from build123d import *

# Parameters (mm, degrees)
BOSS_EXTRU_1_CORPS_DEPTH    = 110
CONG_1_R                    = 1.5
CONG_2_R                    = 0.4
CONG_4_R                    = 1
CONG_1_OF_SYM_TRIE_BRAS_R   = 1.5
CONG_2_OF_SYM_TRIE_BRAS_R   = 0.4
CONG_4_OF_SYM_TRIE_BRAS_R   = 1
SYM_TRIE_BRAS_DOUBLE_DEPTH  = 110
APR_S_TARODAGE_M6_R         = 3
ENL_V_MAT_FILETAGE_M6_DEPTH = 111.905365064


# Read off the part's stored shape, not the designer's step: Symétrie Bras double
with BuildPart() as part:
    # Esquisse4 → Boss.-Extru.1 Corps (new body)
    with BuildSketch(Plane(origin=(0, 0, 0), x_dir=(1, 0, 0), z_dir=(0, 1, 0))):
        Polygon((0, 0), (-4.5, 0), (-4.5, 3.625), (-6.875, 6), (-8.5, 6), (-8.5, 3), (-9.5, 3), (-9.5, 3.5), (-10, 3.5), (-10, 10), (-3.5, 10), (-3.5, 9.5), (-3, 9.5), (-3, 8.5), (-6, 8.5), (-6, 6.875), (-3.625, 4.5), (0, 4.5), align=None)
    boss_extru_1_corps = extrude(amount=BOSS_EXTRU_1_CORPS_DEPTH)

    # Congé1
    cong_1_edges = [part.edges().sort_by_distance(p)[0] for p in [
        (-10, 55, -10),
    ]]
    fillet(cong_1_edges, radius=CONG_1_R)

    # Congé2
    cong_2_edges = [part.edges().sort_by_distance(p)[0] for p in [
        (-8.5, 55, -6),
        (-6, 55, -8.5),
    ]]
    fillet(cong_2_edges, radius=CONG_2_R)

    # Congé4
    cong_4_edges = [part.edges().sort_by_distance(p)[0] for p in [
        (-4.5, 55, -3.625),
        (-6.875, 55, -6),
        (-6, 55, -6.875),
        (-3.625, 55, -4.5),
    ]]
    fillet(cong_4_edges, radius=CONG_4_R)

    # Symétrie Bras: Boss.-Extru.1 Corps across plane
    add(boss_extru_1_corps.mirror(Plane(origin=(0, 110, -4.5), x_dir=(0, 0, 1), z_dir=(-1, 0, 0))))

    # Congé1 of Symétrie Bras
    cong_1_of_sym_trie_bras_edges = [part.edges().sort_by_distance(p)[0] for p in [
        (10, 55, -10),
    ]]
    fillet(cong_1_of_sym_trie_bras_edges, radius=CONG_1_OF_SYM_TRIE_BRAS_R)

    # Congé2 of Symétrie Bras
    cong_2_of_sym_trie_bras_edges = [part.edges().sort_by_distance(p)[0] for p in [
        (8.5, 55, -6),
        (6, 55, -8.5),
    ]]
    fillet(cong_2_of_sym_trie_bras_edges, radius=CONG_2_OF_SYM_TRIE_BRAS_R)

    # Congé4 of Symétrie Bras
    cong_4_of_sym_trie_bras_edges = [part.edges().sort_by_distance(p)[0] for p in [
        (4.5, 55, -3.625),
        (6.875, 55, -6),
        (6, 55, -6.875),
        (3.625, 55, -4.5),
    ]]
    fillet(cong_4_of_sym_trie_bras_edges, radius=CONG_4_OF_SYM_TRIE_BRAS_R)

    # Symétrie Bras double outline → Symétrie Bras double (add)
    with BuildSketch(Plane(origin=(0, 0, 0), x_dir=(1, 0, 0), z_dir=(0, 1, 0))):
        with BuildLine():
            ThreePointArc((7.289213562, -6), (6.90653013, -5.923879533), (6.582106781, -5.707106781))
            Line((6.582106781, -5.707106781), (4.792893219, -3.917893219))
            ThreePointArc((4.792893219, -3.917893219), (4.576120467, -3.59346987), (4.5, -3.210786438))
            Line((4.5, -3.210786438), (4.5, 0))
            Line((4.5, 0), (-4.5, 0))
            Line((-4.5, 0), (-4.5, -3.210786438))
            ThreePointArc((-4.5, -3.210786438), (-4.576120467, -3.59346987), (-4.792893219, -3.917893219))
            Line((-4.792893219, -3.917893219), (-6.582106781, -5.707106781))
            ThreePointArc((-6.582106781, -5.707106781), (-6.90653013, -5.923879533), (-7.289213562, -6))
            Line((-7.289213562, -6), (-8.1, -6))
            ThreePointArc((-8.1, -6), (-8.382842712, -5.882842712), (-8.5, -5.6))
            Line((-8.5, -5.6), (-8.5, -3))
            Line((-8.5, -3), (-9.5, -3))
            Line((-9.5, -3), (-9.5, -3.5))
            Line((-9.5, -3.5), (-10, -3.5))
            Line((-10, -3.5), (-10, -8.5))
            ThreePointArc((-10, -8.5), (-9.560660172, -9.560660172), (-8.5, -10))
            Line((-8.5, -10), (-3.5, -10))
            Line((-3.5, -10), (-3.5, -9.5))
            Line((-3.5, -9.5), (-3, -9.5))
            Line((-3, -9.5), (-3, -8.5))
            Line((-3, -8.5), (-5.6, -8.5))
            ThreePointArc((-5.6, -8.5), (-5.882842712, -8.382842712), (-6, -8.1))
            Line((-6, -8.1), (-6, -7.289213562))
            ThreePointArc((-6, -7.289213562), (-5.923879533, -6.90653013), (-5.707106781, -6.582106781))
            Line((-5.707106781, -6.582106781), (-3.917893219, -4.792893219))
            ThreePointArc((-3.917893219, -4.792893219), (-3.59346987, -4.576120467), (-3.210786438, -4.5))
            Line((-3.210786438, -4.5), (3.210786438, -4.5))
            ThreePointArc((3.210786438, -4.5), (3.59346987, -4.576120467), (3.917893219, -4.792893219))
            Line((3.917893219, -4.792893219), (5.707106781, -6.582106781))
            ThreePointArc((5.707106781, -6.582106781), (5.923879533, -6.90653013), (6, -7.289213562))
            Line((6, -7.289213562), (6, -8.1))
            ThreePointArc((6, -8.1), (5.882842712, -8.382842712), (5.6, -8.5))
            Line((5.6, -8.5), (3, -8.5))
            Line((3, -8.5), (3, -9.5))
            Line((3, -9.5), (3.5, -9.5))
            Line((3.5, -9.5), (3.5, -10))
            Line((3.5, -10), (8.5, -10))
            ThreePointArc((8.5, -10), (9.560660172, -9.560660172), (10, -8.5))
            Line((10, -8.5), (10, -3.5))
            Line((10, -3.5), (9.5, -3.5))
            Line((9.5, -3.5), (9.5, -3))
            Line((9.5, -3), (8.5, -3))
            Line((8.5, -3), (8.5, -5.6))
            ThreePointArc((8.5, -5.6), (8.382842712, -5.882842712), (8.1, -6))
            Line((8.1, -6), (7.289213562, -6))
        make_face()
    extrude(amount=SYM_TRIE_BRAS_DOUBLE_DEPTH)

    # Après tarodage M6 → Enlèv. mat.-Filetage M6 (cut, through all)
    with BuildSketch(Plane.XZ):
        with Locations(Location((0, 0, 0), (0, 0, 270))):
            Circle(APR_S_TARODAGE_M6_R)
    extrude(amount=-ENL_V_MAT_FILETAGE_M6_DEPTH, mode=Mode.SUBTRACT)


solid = part.part
Input: part model. Units: mm. Frame: model coordinates. A direction names the side the tool comes from. Give positions to 0.01 mm unless a question says otherwise; leave off trailing zeros. Order: outer loops, then holes, each group sorted by start corner. A loop starts at its lowest first (then second) coordinate and runs counter-clockwise, first axis right, second up. Notation, with made-up numbers: (3, 46.25) - (28, 46.25) arc R27 cw to (28, 79.25) - close; hole circle Ø4 at (-31, -22). An arc over 180 degrees is marked (long way). Answer as a JSON object with one key per item and string values. Group by question number.
Q1. Set-up query: faces 1 (the face through (10, 54, -6)), 2 (the face through (-4.825, 54.23, 5.7)). Return all of +Z, -Z, +X, -X, +Y, -Y with unobstructed straight access to the full face (end or side cutting, diameter ignored); none if empty.
Q2. Cut plane B-B, the plane z = 0. Output: boundary loops of the cut face in (x, y).
Q3. Mould query, pull axis X, two halves, no side actions, for faces 3 (the face through (2.1, 110, -2.4)), 4 (the face through (-10, 54, 6)), 5 (the face through (4.825, 54.23, -5.7)). Classes: pulls with the +X half, pulls with the -X half, needs draft (parallel to the pull), parting line crosses it, or undercut.
Q4. Cut plane A-A, the plane x = 0. Output: boundary loops of the cut face in (y, z).
Q5. Line query: probe 1 along X at (y, z) = (85, 0); probe 2 along Z at (x, y) = (-0.25, 96.5); probe 3 along Z at (x, y) = (8.75, 103). Output: solid intervals per line, ascending.
Q6. First-contact query: pin 1 Ø0.6 at (y, z) = (78, -9.5) entering from -X; pin 2 Ø1.5 at (x, y) = (-2.5, 47.5) entering from -Z; pin 3 Ø0.6 at (x, y) = (3, 79) entering from +Z. Flat tips, straight axial feed; report the tip coordinate or a pass-through.
Results:
{
 "1": {"face 1": "+Z, -Z, +X, +Y, -Y", "face 2": "+Y, -Y"},
 "2": {"outline": "(-4.5, 0) - (-3, 0) - (-3, 110) - (-4.5, 110) - close; (3, 0) - (4.5, 0) - (4.5, 110) - (3, 110) - close"},
 "3": {"face 3": "needs draft", "face 4": "pulls with the -X half", "face 5": "undercut"},
 "4": {"outline": "(0, -4.5) - (110, -4.5) - (110, -3) - (0, -3) - close; (0, 3) - (110, 3) - (110, 4.5) - (0, 4.5) - close"},
 "5": {"probe 1": "-4.5 to -3, 3 to 4.5", "probe 2": "-4.5 to -2.99, 2.99 to 4.5", "probe 3": "-9.98 to -3, 3 to 9.98"},
 "6": {"pin 1": "x = -9.83", "pin 2": "z = -9.5", "pin 3": "z = 9.5"}
}
